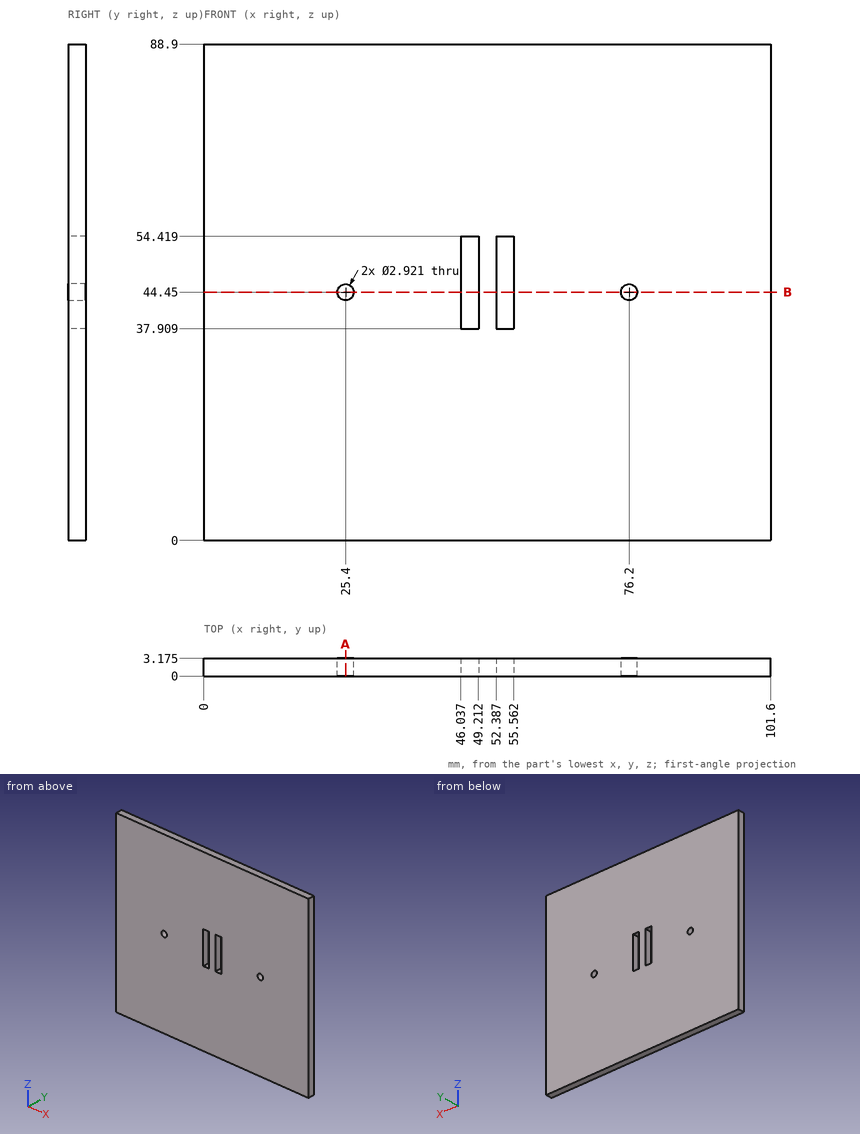
Geometry check sheet. Reference: drawing and pictorial views, mm from the part's lowest x, y, z. Coordinates: 2 decimals unless noted, no trailing zeros. Order: outer loops, then holes, each group sorted by start corner. A loop starts at its lowest first (then second) coordinate and runs counter-clockwise, first axis right, second up.
1. Sectioned sample at A-A, the plane x = 25.4. Record the cut outline in (y, z) (1 decimal), and give its area (3 significant figures).
Results found:
outline: (0, 0) - (3.2, 0) - (3.2, 43) - (0, 43) - close; (0, 45.9) - (3.2, 45.9) - (3.2, 88.9) - (0, 88.9) - close
area: 273 mm2
2. Sectioned sample at B-B, the plane z = 44.45. Record the cut outline in (x, y) (1 decimal).
Results found:
outline: (0, 0) - (23.9, 0) - (23.9, 3.2) - (0, 3.2) - close; (26.9, 0) - (46, 0) - (46, 3.2) - (26.9, 3.2) - close; (49.2, 0) - (52.4, 0) - (52.4, 3.2) - (49.2, 3.2) - close; (55.6, 0) - (74.7, 0) - (74.7, 3.2) - (55.6, 3.2) - close; (77.7, 0) - (101.6, 0) - (101.6, 3.2) - (77.7, 3.2) - close
3. Scan lines: line 1 (X direction, y = 1.9, z = 44.45); line 2 (Z direction, x = 76.2, y = 2.3). Record each from-to range of solid material in increasing order.
Results found:
line 1: x = 0 to 23.94, 26.86 to 46.04, 49.21 to 52.39, 55.56 to 74.74, 77.66 to 101.6
line 2: z = 0 to 42.99, 45.91 to 88.9
